from build123d import *

# Parameters (mm, degrees)
SKETCH1_W               = 70
SKETCH1_H               = 80
BOSS_EXTRUDE1_DEPTH     = 70
SKETCH2_W               = 45
SKETCH2_H               = 40
CUT_EXTRUDE1_DEPTH      = 70
CUT_EXTRUDE2_DEPTH      = 112.915146428
CUT_EXTRUDE2_DEPTH_BACK = 112.915146428
BOSS_EXTRUDE2_DEPTH     = 20
SKETCH5_R               = 17.5
CUT_EXTRUDE3_DEPTH      = 20


with BuildPart() as part:
    # Sketch1 → Boss-Extrude1 (new body)
    with BuildSketch(Plane.XY):
        Rectangle(SKETCH1_W, SKETCH1_H)
    extrude(amount=BOSS_EXTRUDE1_DEPTH)

    # Sketch2 → Cut-Extrude1 (cut)
    with BuildSketch(Plane.XY.offset(70)):
        with Locations((12.5, 0)):
            Rectangle(SKETCH2_W, SKETCH2_H)
    extrude(amount=-CUT_EXTRUDE1_DEPTH, mode=Mode.SUBTRACT)

    # Sketch3 → Cut-Extrude2 (cut, two sides: drawn at the far end of the back side and taken through both)
    with BuildSketch(Plane(origin=(0, 40, 0), x_dir=(1, 0, 0), z_dir=(0, 1, 0)).offset(-CUT_EXTRUDE2_DEPTH_BACK)):
        with BuildLine():
            Line((-35, -55), (-35, -15))
            ThreePointArc((-35, -15), (-15, -35), (-35, -55))
        make_face()
    extrude(amount=CUT_EXTRUDE2_DEPTH + CUT_EXTRUDE2_DEPTH_BACK, mode=Mode.SUBTRACT)

    # Sketch4 → Boss-Extrude2 (add)
    with BuildSketch(Plane(origin=(35, 0, 0), x_dir=(0, 0, -1), z_dir=(1, 0, 0))):
        with BuildLine():
            Line((-70, 40), (-70, 80))
            ThreePointArc((-70, 80), (-35, 115), (0, 80))
            Line((0, 80), (0, 40))
            Line((0, 40), (-70, 40))
        make_face()
    extrude(amount=-BOSS_EXTRUDE2_DEPTH)

    # Sketch5 → Cut-Extrude3 (cut)
    with BuildSketch(Plane(origin=(35, 0, 0), x_dir=(0, 0, -1), z_dir=(1, 0, 0))):
        with Locations((-35, 80)):
            Circle(SKETCH5_R)
    extrude(amount=-CUT_EXTRUDE3_DEPTH, mode=Mode.SUBTRACT)


solid = part.part
Read the model definition and answer for the solid it produces. Units are mm, in the model's axes. A direction names the side the tool comes from. Coordinates: 2 decimals unless noted, no trailing zeros. Order: outer loops, then holes, each group sorted by start corner. A loop starts at its lowest first (then second) coordinate and runs counter-clockwise, first axis right, second up. Notation, with made-up numbers: M 0,-35 L 33,-35 A4 cw 33,-30 Z; hole C 79.25,59 d11. An arc over 180 degrees is marked long. Put each result on its own line as item: value. Start each with the question number.
Item 1: Section C-C, the plane x = 5.5 is taken. Determine the outline of the cut face in (y, z), plus the area to 3 significant figures.
Item 2: For faces 4 (the face through (0, 21, 0)), 5 (the face through (-10, 0, 35)), 6 (the face through (15, 61, 35)), determine the directions among +Z, -Z, +X, -X, +Y, -Y from which every point of the face is accessible in a straight line to the end or side of a thin tool.
Item 3: Section B-B, the plane z = 35 is taken. Determine the outline of the cut face in (x, y), plus the area to 3 significant figures.
Item 4: The mould has two halves that part along Y. Classify faces 1 (the face through (-5, 40, 35)), 2 (the face through (12, -20, 35)), 3 (the face through (-15, -1, 35)): +Y half, -Y half, draft (parallel to the pull), parting line (faces both ways), or undercut.
Item 5: Given pin 1 Ø15 at (x, z) = (-19, 26) entering from +Y; pin 2 Ø22.5 at (x, z) = (23.5, 38.5) entering from +Y, each flat-ended and moving along its own axis, determine where each tip first touches the part or whether it passes through.
Item 6: Section D-D, the plane y = 35.5 is taken. Determine the outline of the cut face in (x, z), plus the area to 3 significant figures.
Item 7: Section A-A, the plane x = 23 is taken. Determine the outline of the cut face in (y, z).
Item 8: Consider probe 1 along Y at (x, z) = (23, 35); probe 2 along Y at (x, z) = (13, 42); probe 3 along Y at (x, z) = (32.5, 23). Determine where each line is inside the solid, lowest interval first. Write a range as [from, to].
Computed:
1. outline: M -40,0 L -20,0 L -20,70 L -40,70 Z; M 20,0 L 40,0 L 40,70 L 20,70 Z
1. area: 2,800 mm2
2. face 4: -Z, +X, -X, +Y, -Y
2. face 5: +Z, -Z, +X
2. face 6: +Z, -Z, -X, +Y
3. outline: M -15,-40 L 35,-40 L 35,-20 L -10,-20 L -10,20 L 35,20 L 35,62.5 L 15,62.5 L 15,40 L -15,40 Z; M 15,97.5 L 35,97.5 L 35,115 L 15,115 Z
3. area: 3,000 mm2
4. face 1: +Y half
4. face 2: undercut
4. face 3: draft
5. pin 1: stops at y = 40
5. pin 2: stops at y = 115
6. outline: M -35,0 L 35,0 L 35,70 L -35,70 L -35,55 A20 cw -35,15 Z
6. area: 4,270 mm2
7. outline: M -40,0 L -20,0 L -20,70 L -40,70 Z; M 20,0 L 80,0 A35 ccw 80,70 L 20,70 Z; hole C 80,35 d35
8. probe 1: y = [-40, -20], [20, 62.5], [97.5, 115]
8. probe 2: y = [-40, -20], [20, 40]
8. probe 3: y = [-40, -20], [20, 67.26], [92.74, 112.88]
